Input: dimensioned drawing with shaded views. Units: mm. Origin: part minimum x, y, z. A direction names the side the tool comes from. Give positions to 0.01 mm unless a question says otherwise; leave off trailing zeros. Order: outer loops, then holes, each group sorted by start corner. A loop starts at its lowest first (then second) coordinate and runs counter-clockwise, first axis right, second up. Notation, with made-up numbers: (46.25, 71.5) - (63.25, 71.5) arc R4 ccw to (63.25, 76.5) - close; hole circle Ø6 at (22.5, 22.5). An arc over 180 degrees is marked (long way). Use a Markdown table: item, result.
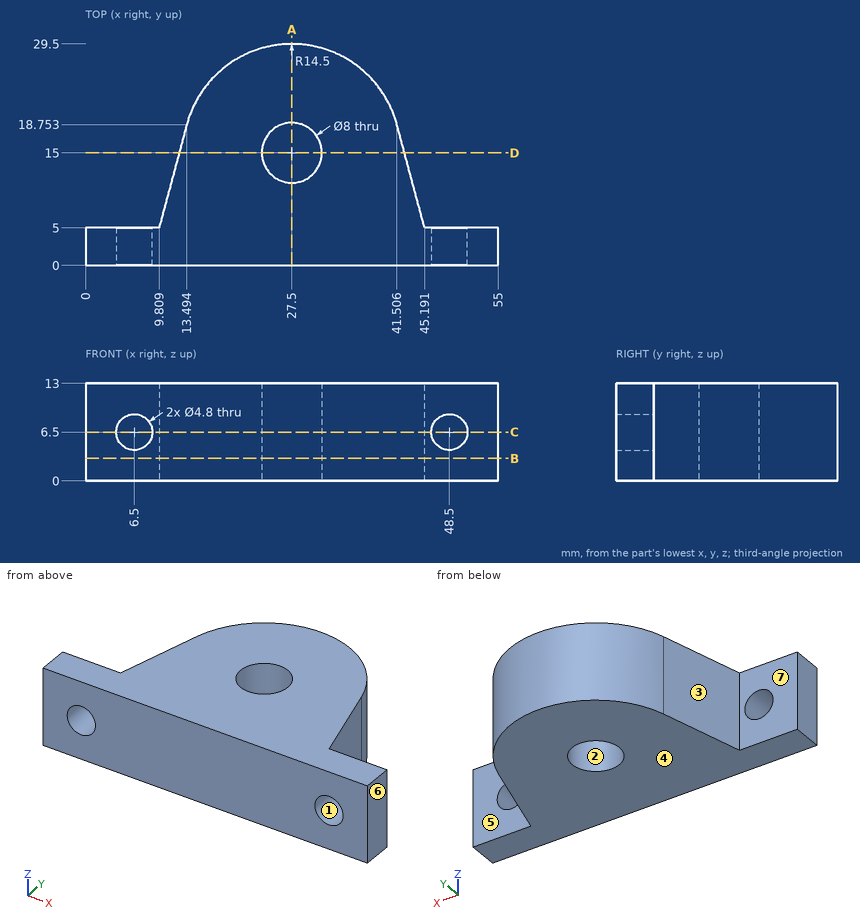
1. Material intervals for line 1 along Y through (x, z) = (50.5, 11); line 2 along X through (y, z) = (18.5, 7); line 3 along X through (y, z) = (11.5, 7.5), sorted ascending.
Response:
| item | result |
|---|---|
| line 1 | y = 0 to 5 |
| line 2 | x = 13.43 to 25.56, 29.44 to 41.57 |
| line 3 | x = 11.55 to 25.56, 29.44 to 43.45 |
2. Section query A-A (x = 27.5). Return loops of the section in (y, z), then the cut area to 4 significant figures.
Response:
| item | result |
|---|---|
| outline | (0, 0) - (11, 0) - (11, 13) - (0, 13) - close; (19, 0) - (29.5, 0) - (29.5, 13) - (19, 13) - close |
| area | 279.5 mm^2 |
3. Mould query, pull axis X, two halves, no side actions, for the marked faces 1, 2, 3 and 4. Classes: pulls with the +X half, pulls with the -X half, needs draft (parallel to the pull), parting line crosses it, or undercut.
Response:
| item | result |
|---|---|
| face 1 | undercut |
| face 2 | undercut |
| face 3 | pulls with the -X half |
| face 4 | needs draft |
4. Section query D-D (y = 15). Return loops of the section in (x, z).
Response:
| item | result |
|---|---|
| outline | (12.49, 0) - (23.5, 0) - (23.5, 13) - (12.49, 13) - close; (31.5, 0) - (42.51, 0) - (42.51, 13) - (31.5, 13) - close |
5. Section query B-B (z = 3). Return loops of the section in (x, y).
Response:
| item | result |
|---|---|
| outline | (0, 0) - (55, 0) - (55, 5) - (45.19, 5) - (41.51, 18.75) arc R14.5 ccw to (13.49, 18.75) - (9.81, 5) - (0, 5) - close; hole circle Ø8 at (27.5, 15) |
6. Section query C-C (z = 6.5). Return loops of the section in (x, y).
Response:
| item | result |
|---|---|
| outline | (0, 0) - (4.1, 0) - (4.1, 5) - (0, 5) - close; (8.9, 0) - (46.1, 0) - (46.1, 5) - (45.19, 5) - (41.51, 18.75) arc R14.5 ccw to (13.49, 18.75) - (9.81, 5) - (8.9, 5) - close; (50.9, 0) - (55, 0) - (55, 5) - (50.9, 5) - close; hole circle Ø8 at (27.5, 15) |
7. Set-up query: the marked faces 5, 6 and 7. Return all of +Z, -Z, +X, -X, +Y, -Y with unobstructed straight access to the full face (end or side cutting, diameter ignored); none if empty.
Response:
| item | result |
|---|---|
| face 5 | +Z, -Z, +X, +Y |
| face 6 | +Z, -Z, +X, +Y, -Y |
| face 7 | +Z, -Z, -X, +Y |
8. Pin query (flat end, axial travel): pin 1 (3 mm diameter, centred on x = 3.5, z = 3.5, fed in from +Y); pin 2 (4 mm diameter, centred on y = 26.5, z = 7, fed in from -X); pin 3 (4 mm diameter, centred on y = 7.5, z = 10.5, fed in from +X); pin 4 (12 mm diameter, centred on x = 49.5, y = 15, fed in from +Z). Return the tip coordinate at first contact, or that it passes through.
Response:
| item | result |
|---|---|
| pin 1 | stops at y = 5 |
| pin 2 | stops at x = 16.55 |
| pin 3 | stops at x = 45.06 |
| pin 4 | passes through |
